Job drawing, mm, ordinate dimensions from the low corner. One solid piece. A direction names the side the tool comes from. Give positions to 0.01 mm unless a question says otherwise; leave off trailing zeros. Loops run counter-clockwise (first coordinate to the right, second up) from the corner with the lowest first, then second, coordinate; pieces in that order, holes last. Notation, with made-up numbers: (-36.5, -36.5) -> (-2.5, -36.5) arc R19 ccw to (-2.5, -21.5) -> close; hole circle Ø7 at (40.25, 85.5). An arc over 180 degrees is marked (long way). Use one line per item in the form item = value.
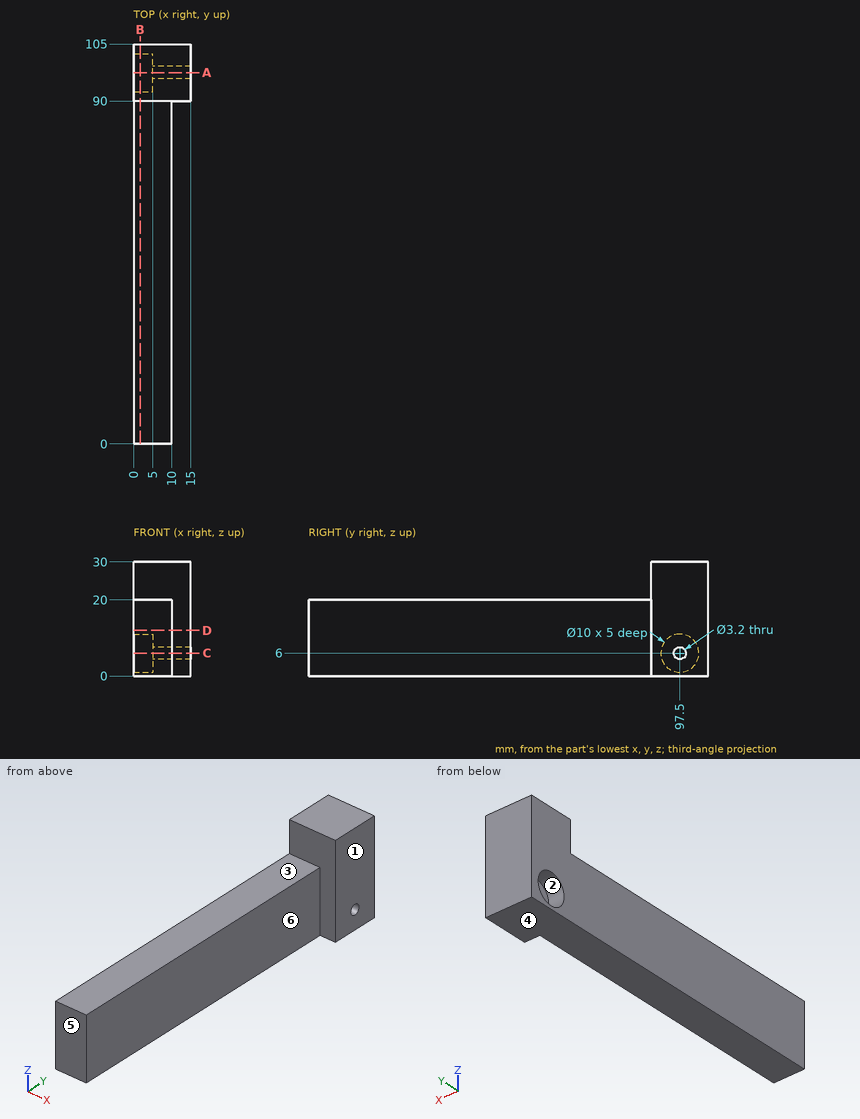
1. Cut at C-C, the plane z = 6. Write the cut outline in (x, y).
Result sheet:
outline = (0, 0) -> (10, 0) -> (10, 90) -> (15, 90) -> (15, 95.9) -> (5, 95.9) -> (5, 92.5) -> (0, 92.5) -> close; (0, 102.5) -> (5, 102.5) -> (5, 99.1) -> (15, 99.1) -> (15, 105) -> (0, 105) -> close
2. Drop flat-ended pins along their axis: P1, Ø3, axis at x = 5.5, y = 31.5, coming from the +Z side; P2, Ø6, axis at y = 35.5, z = 9, coming from the +X side; P3, Ø6, axis at y = 97.5, z = 6, coming from the -X side. Give the stop position or say it passes through.
Result sheet:
P1 = 20
P2 = 10
P3 = 5
3. Tool access for the marked faces 5 and 6: list every direction of +Z, -Z, +X, -X, +Y, -Y with a clear straight run to the whole face (end or side of a thin tool).
Result sheet:
face_5 = +Z, -Z, +X, -X, -Y
face_6 = +Z, -Z, +X, -Y
4. Cut at A-A, the plane y = 97.5. Write the cut outline in (x, z).
Result sheet:
outline = (0, 0) -> (15, 0) -> (15, 4.4) -> (5, 4.4) -> (5, 1) -> (0, 1) -> close; (0, 11) -> (5, 11) -> (5, 7.6) -> (15, 7.6) -> (15, 30) -> (0, 30) -> close
5. Cut at B-B, the plane x = 1.75. Write the cut outline in (y, z).
Result sheet:
outline = (0, 0) -> (105, 0) -> (105, 30) -> (90, 30) -> (90, 20) -> (0, 20) -> close; hole circle Ø10 at (97.5, 6)
6. Cut at D-D, the plane z = 12. Write the cut outline in (x, y), then the cut area to 4 significant figures.
Result sheet:
outline = (0, 0) -> (10, 0) -> (10, 90) -> (15, 90) -> (15, 105) -> (0, 105) -> close
area = 1,125 mm^2
7. Mould opens along Z. For the marked faces 1, 2, 3 and 4 say: pulls with the +Z half, pulls with the -Z half, needs draft (parallel to the pull), parting line crosses it, or undercut.
Result sheet:
face_1 = needs draft
face_2 = undercut
face_3 = pulls with the +Z half
face_4 = pulls with the -Z half
8. Drill centre lines: line 1 (Y direction, x = 9.25, z = 6); line 2 (Z direction, x = 12.25, y = 97.5); line 3 (Y direction, x = 11.25, z = 6). Where is each one in solid material? Low to high.
Result sheet:
line_1 = 0 to 95.9, 99.1 to 105
line_2 = 0 to 4.4, 7.6 to 30
line_3 = 90 to 95.9, 99.1 to 105
